```python
from build123d import *

# Parameters (mm, degrees)
SKETCH1_W               = 38.1
SKETCH1_H               = 38.1
BOSS_EXTRUDE1_DEPTH     = 442.976
CUT_EXTRUDE1_DEPTH      = 446.019380562
CUT_EXTRUDE2_DEPTH      = 446.019380562
CUT_EXTRUDE2_DEPTH_BACK = 446.019380562


with BuildPart() as part:
    # Sketch1 → Boss-Extrude1 (new body)
    with BuildSketch(Plane(origin=(0, 0, 0), x_dir=(0, 0, -1), z_dir=(1, 0, 0))):
        Rectangle(SKETCH1_W, SKETCH1_H)
    extrude(amount=BOSS_EXTRUDE1_DEPTH)

    # Sketch2 → Cut-Extrude1 (cut, through all)
    with BuildSketch(Plane.XY.offset(19.05)):
        Polygon((442.976, -19.05), (408.36839663, 19.05), (442.976, 19.05), align=None)
    extrude(amount=-CUT_EXTRUDE1_DEPTH, mode=Mode.SUBTRACT)

    # Sketch3 → Cut-Extrude2 (cut, two sides: drawn at the far end of the back side and taken through both)
    with BuildSketch(Plane.XY.offset(19.05).offset(-CUT_EXTRUDE2_DEPTH_BACK)):
        Polygon((0, 19.05), (0, -0.569448187), (1.811202923, 19.05), align=None)
        Polygon((0, -0.569448187), (1.811202923, 19.05), (10.756321618, 9.121476911), align=None)
    extrude(amount=CUT_EXTRUDE2_DEPTH + CUT_EXTRUDE2_DEPTH_BACK, mode=Mode.SUBTRACT)


solid = part.part
```
Design review of the part built by this model. Coordinates are the model's own, in mm. A direction names the side the tool comes from. Round coordinates to 2 decimals unless told otherwise and drop trailing zeros. Write each loop counter-clockwise with the first axis right and the second up, starting at its lowest first coordinate (ties: lowest second). Pieces come first, ordered by that corner, then holes.
Item 1: We need section B-B on y = -10.5. Write out the cut boundary in (x, z).
Item 2: The part is to be moulded in two halves that separate along Y. For faces 1 (the flat face through (5.45, 4.34, -0.27)), 2 (the flat face through (202, 19.05, 0)), 3 (the flat face through (0, -10, 0)), say which applies: +Y half, -Y half, draft (parallel to the pull), parting line (faces both ways), or undercut.
Item 3: For faces 4 (the flat face through (6.221, 14.155, -0.267)), 5 (the flat face through (218, 0, -19.05)), list the 3-axis set-ups (+Z, -Z, +X, -X, +Y, -Y) from which the entire face can be reached by the end or side of a thin tool; tool diameter is ignored.
Item 4: We need section A-A on z = 13.5. Write out the cut boundary in (x, y).
Item 5: We need section C-C on y = 13. Write out the cut boundary in (x, z).
Item 6: For probe 1 along X at (y, z) = (16, -13.5); probe 2 along X at (y, z) = (1.5, -12), list the stretches that pass through material, from the lowest coordinate up.
Item 7: Clearance check with flat-ended pins moving along their axes: pin 1 Ø8 at (y, z) = (14.5, -3) entering from +X; pin 2 Ø4 at (y, z) = (-2.5, 4) entering from +X; pin 3 Ø1.5 at (y, z) = (-9.5, -9.5) entering from +X. State where each tip first meets the part, or that it passes through.
Returned:
1. outline: (0, -19.05) - (435.21, -19.05) - (435.21, 19.05) - (0, 19.05) - close
2. face 1: undercut
2. face 2: +Y half
2. face 3: draft
3. face 4: +Z, -Z, -X
3. face 5: -Z, +X, -X, +Y, -Y
4. outline: (0, -19.05) - (442.98, -19.05) - (408.37, 19.05) - (1.81, 19.05) - (10.76, 9.12) - (0, -0.57) - close
5. outline: (7.26, -19.05) - (413.86, -19.05) - (413.86, 19.05) - (7.26, 19.05) - close
6. probe 1: x = 4.56 to 411.14
6. probe 2: x = 2.3 to 424.31
7. pin 1: stops at x = 416.13
7. pin 2: stops at x = 429.76
7. pin 3: stops at x = 434.98
